Print and shaded views of the part. All mm, measured from the part's lowest x, y and z. A direction names the side the tool comes from. Give positions to 0.01 mm unless a question says otherwise; leave off trailing zeros. Write each loop counter-clockwise with the first axis right and the second up, starting at its lowest first coordinate (ties: lowest second). Pieces come first, ordered by that corner, then holes. Notation, with made-up numbers: M 88.25,72 L 102.25,72 A15 ccw 102.25,98 Z; hole C 66,-28.5 d1. An arc over 180 degrees is marked long. One line per question, with ' | ' between items. Start each with the question number.
1. Flat gauge pins, fed straight in: pin 1 (8 mm diameter, centred on x = 17.5, z = 11.5, fed in from -Y); pin 2 (4 mm diameter, centred on y = 22.5, z = 4.5, fed in from -X); pin 3 (1.5 mm diameter, centred on y = 8.5, z = 2.5, fed in from -X). Where does each tip first touch, or does it go through?
2. Cut at B-B, the plane x = 22.5. Write the cut outline in (y, z), then the cut area to 3 significant figures.
3. Cut at A-A, the plane z = 6.25. Write the cut outline in (x, y).
4. Pull direction X, two halves, no side cores. Call the marked faces 1, 2 and 3: released by +X, released by -X, zero draft, split by the parting line, or undercut.
5. Wall check: L1, parallel to X at y = 35, z = 7.5; L2, parallel to Z at x = 22.5, y = 32.25; L3, parallel to X at y = 25.5, z = 11.5. Give the ranges that are in metal, low to high.
6. Cut at C-C, the plane z = 1.75. Write the cut outline in (x, y).
7. Which spindle directions (+Z, -Z, +X, -X, +Y, -Y) get a long thin tool onto all of the face, cutting with end or side? Do the marked faces 4 and 5. Say none if no direction does.
8. Cut at D-D, the plane x = 66. Write the cut outline in (y, z), then the cut area to 3 significant figures.
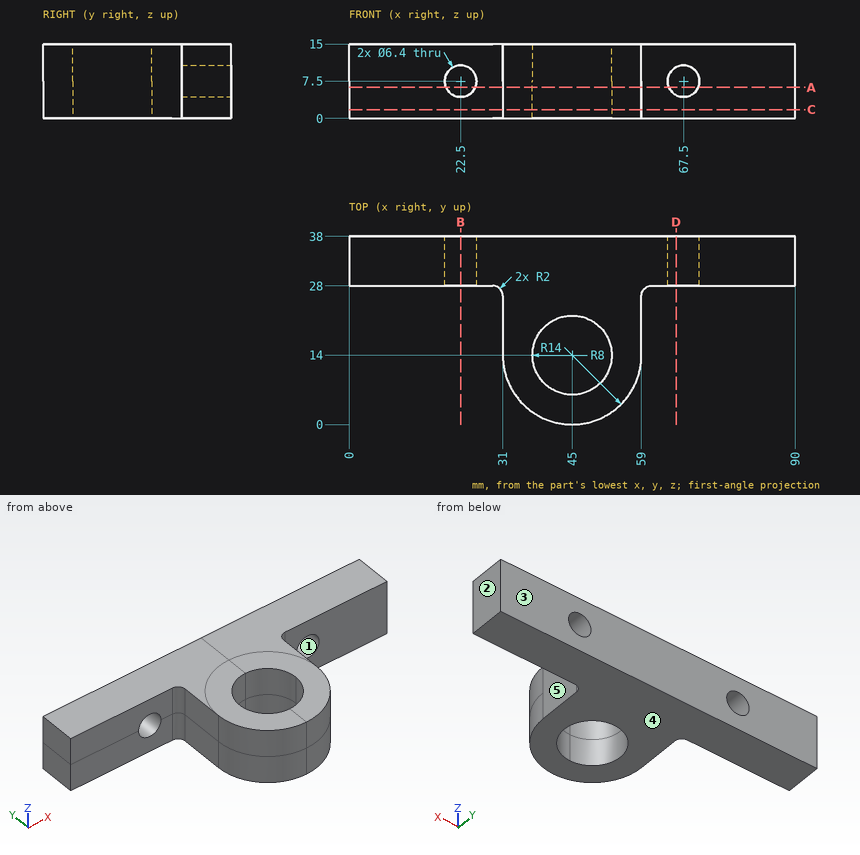
Here are the results:
1) pin 1: y = 28 | pin 2: x = 31 | pin 3: x = 31.83
2) outline: M 28,0 L 38,0 L 38,4.3 L 28,4.3 Z; M 28,10.7 L 38,10.7 L 38,15 L 28,15 Z | area: 86.0 mm^2
3) outline: M 0,28 L 19.55,28 L 19.55,38 L 0,38 Z; M 25.45,28 L 29,28 A2 cw 31,26 L 31,14 A14 ccw 59,14 L 59,26 A2 cw 61,28 L 64.55,28 L 64.55,38 L 25.45,38 Z; M 70.45,28 L 90,28 L 90,38 L 70.45,38 Z; hole C 45,14 d16
4) face 1: undercut | face 2: released by +X | face 3: zero draft
5) L1: 0 to 19.3, 25.7 to 64.3, 70.7 to 90 | L2: 0 to 4.3, 10.7 to 15 | L3: 31 to 59
6) outline: M 0,28 L 29,28 A2 cw 31,26 L 31,14 A14 ccw 59,14 L 59,26 A2 cw 61,28 L 90,28 L 90,38 L 0,38 Z; hole C 45,14 d16
7) face 4: -Z, +X, -X, +Y, -Y | face 5: +Z, -Z, +X, -Y
8) outline: M 28,0 L 38,0 L 38,4.67 L 28,4.67 Z; M 28,10.33 L 38,10.33 L 38,15 L 28,15 Z | area: 93.5 mm^2
